Input: part model. Units: mm. Frame: model coordinates. A direction names the side the tool comes from. Coordinates: 2 decimals unless noted, no trailing zeros. Order: outer loops, then holes, each group sorted by start corner. A loop starts at its lowest first (then second) coordinate and runs counter-clockwise, first axis right, second up. Notation, with made-up numbers: (-36, -21) -> (-20, -21) arc R10 ccw to (-20, -12) -> close; hole circle Ø9 at (89, 65.5). An arc over 180 degrees is marked (long way). Answer as CSV lines item,"result".
from build123d import *

# Parameters (mm, degrees)
SKETCH1_R           = 51
SKETCH1_R_2         = 50
EXTRUDE_THIN1_DEPTH = 100
SKETCH1_2_R         = 50
BOSS_EXTRUDE1_DEPTH = 1
LPATTERN1_COUNT     = 2
LPATTERN1_PITCH     = 99
SKETCH3_R           = 5
CUT_EXTRUDE1_DEPTH  = 101


with BuildPart() as part:
    # Sketch1 → Extrude-Thin1 (new body)
    with BuildSketch(Plane(origin=(0, 0, 0), x_dir=(1, 0, 0), z_dir=(0, 1, 0))):
        Circle(SKETCH1_R)
        Circle(SKETCH1_R_2, mode=Mode.SUBTRACT)
    extrude(amount=EXTRUDE_THIN1_DEPTH)

    # Sketch1<2> → Boss-Extrude1 (add)
    with BuildSketch(Plane(origin=(0, 0, 0), x_dir=(1, 0, 0), z_dir=(0, 1, 0))):
        Circle(SKETCH1_2_R)
    boss_extrude1 = extrude(amount=BOSS_EXTRUDE1_DEPTH)

    # LPattern1: Boss-Extrude1 ×2
    with Locations(*[(0, i * LPATTERN1_PITCH, 0) for i in range(1, LPATTERN1_COUNT)]):
        add(boss_extrude1)

    # Sketch3 → Cut-Extrude1 (cut, through all)
    with BuildSketch(Plane.XZ):
        Circle(SKETCH3_R)
    extrude(amount=-CUT_EXTRUDE1_DEPTH, mode=Mode.SUBTRACT)


solid = part.part
1. Cut plane D-D (z = -25). Return the cut outline in (x, y).
Findings:
outline,"(-44.45, 0) -> (44.45, 0) -> (44.45, 100) -> (-44.45, 100) -> close; hole (-43.3, 1) -> (43.3, 1) -> (43.3, 99) -> (-43.3, 99) -> close"
2. Cut plane B-B (x = 0). Return the cut outline in (y, z).
Findings:
outline,"(0, -51) -> (100, -51) -> (100, -5) -> (99, -5) -> (99, -50) -> (1, -50) -> (1, -5) -> (0, -5) -> close; (0, 5) -> (1, 5) -> (1, 50) -> (99, 50) -> (99, 5) -> (100, 5) -> (100, 51) -> (0, 51) -> close"
3. Reachability of faces 1 (the face through (-1, 1, 10)), 2 (the face through (11, 0, -1)) from +Z, -Z, +X, -X, +Y, -Y: full face, straight path, thin tool, end or side. Return the list, or none.
Findings:
face 1,"none"
face 2,"+Z, -Z, +X, -X, -Y"
4. Cut plane A-A (z = 0). Return the cut outline in (x, y), plus the area to 3 significant figures.
Findings:
outline,"(-51, 0) -> (-5, 0) -> (-5, 1) -> (-50, 1) -> (-50, 99) -> (-5, 99) -> (-5, 100) -> (-51, 100) -> close; (5, 0) -> (51, 0) -> (51, 100) -> (5, 100) -> (5, 99) -> (50, 99) -> (50, 1) -> (5, 1) -> close"
area,"380 mm2"
5. Cut plane C-C (x = 43). Return the cut outline in (y, z).
Findings:
outline,"(0, -27.42) -> (100, -27.42) -> (100, 27.42) -> (0, 27.42) -> close; hole (1, -25.51) -> (99, -25.51) -> (99, 25.51) -> (1, 25.51) -> close"
6. Ray query, line 1 along X through (y, z) = (68, 0.5); line 2 along Y through (x, z) = (31, -36). Return the intervals inside material, ascending.
Findings:
line 1,"x = -51 to -50, 50 to 51"
line 2,"y = 0 to 1, 99 to 100"
7. Contact query for flat-ended pins moving along their axis: pin 1 (8 mm diameter, centred on y = 52, z = -14, fed in from +X); pin 2 (2 mm diameter, centred on x = -4, y = 17, fed in from +Z); pin 3 (8 mm diameter, centred on x = 0, z = 0, fed in from +Y); pin 4 (2 mm diameter, centred on x = 9, y = 69, fed in from -Z). Output: stop coordinate, or through.
Findings:
pin 1,"stops at x = 50.01"
pin 2,"stops at z = 50.91"
pin 3,"passes through"
pin 4,"stops at z = -50.37"
8. Mould query, pull axis Z, two halves, no side actions, for faces 3 (the face through (-11.056, 49.3, 49.787)), 4 (the face through (-1.08, 0.49, -4.88)), 5 (the face through (11, 100, -1)). Classes: released by +Z, released by -Z, zero draft, split by the parting line, or undercut.
Findings:
face 3,"split by the parting line"
face 4,"undercut"
face 5,"zero draft"
